Part model, mm, in its own coordinate system. Round coordinates to 2 decimals unless told otherwise and drop trailing zeros. Write each loop counter-clockwise with the first axis right and the second up, starting at its lowest first coordinate (ties: lowest second). Pieces come first, ordered by that corner, then holes. Notation, with made-up numbers: (78.25, 68) -> (121.25, 68) arc R26 cw to (121.25, 105) -> close; hole circle Ø6 at (63, 78.5). An arc over 180 degrees is marked (long way). Return JSON: item names as keys, results as strings. Group by question number.
(1) Saw through at B-B (x = 1.05). List the corners of the cut face in (y, z), plus the area to 3 significant figures.
(2) Drop flat-ended pins along their axis: pin 1 Ø1.7 at (x, y) = (-21, 1.5) entering from +Z; pin 2 Ø2.5 at (x, y) = (-16, 1) entering from -Z; pin 3 Ø5 at (y, z) = (5, 44) entering from -X. Give the stop position or say it passes through.
(3) Drill centre lines: L1, parallel to X at y = 1.25, z = 115.25; L2, parallel to X at y = 0.4, z = 115.25; L3, parallel to X at y = 7, z = 142.5. Where is each one in solid material? Low to high. Write a range as from..to.
(4) Saw through at A-A (y = 3.75). List the corners of the cut face in (x, z), plus the area to 3 significant figures.
(5) Saw through at C-C (z = 115.25). List the corners of the cut face in (x, y).
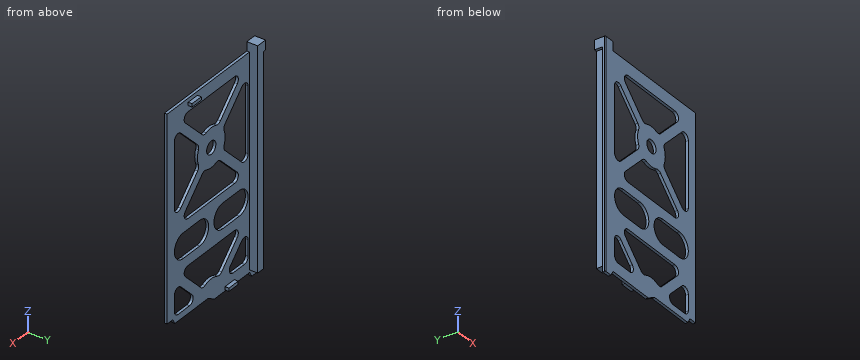
from build123d import *

# Parameters (mm, degrees)
SKETCH1_R           = 5
BOSS_EXTRUDE1_DEPTH = 2.1
SKETCH2_W           = 8.5
SKETCH2_H           = 170.25
BOSS_EXTRUDE2_DEPTH = 6.4
SKETCH3_W           = 162.8
SKETCH3_H           = 6.4
CUT_EXTRUDE1_DEPTH  = 2.1
SKETCH4_W           = 10
SKETCH4_H           = 2.5
BOSS_EXTRUDE3_DEPTH = 3
CHAMFER1_SIZE       = 0.5


with BuildPart() as part:
    # Sketch1 → Boss-Extrude1 (new body)
    with BuildSketch(Plane(origin=(0, 0, 0), x_dir=(1, 0, 0), z_dir=(0, 1, 0))):
        Polygon((-48.95, 0.55), (-48.95, -172.25), (-40.45, -172.25), (-40.45, -165.25), (48.95, -165.25), (48.95, -8), (42.85, -8), (40.540598923, -4), (4.514101615, -4), (-2.414101615, 0), (-40.640598923, 0), (-42.95, 4), (-48.95, 4), align=None)
        with BuildLine():
            Line((-13.76890063, -125.119153161), (-32.121572875, -143.471825407))
            ThreePointArc((-32.121572875, -143.471825407), (-36.480733729, -144.338916412), (-38.95, -140.643398282))
            Line((-38.95, -140.643398282), (-38.95, -89.856601718))
            ThreePointArc((-38.95, -89.856601718), (-36.480733729, -86.161083588), (-32.121572875, -87.028174593))
            Line((-32.121572875, -87.028174593), (-13.76890063, -105.380846839))
            ThreePointArc((-13.76890063, -105.380846839), (-12.679375, -107.403267629), (-12.882100859, -109.691532076))
            ThreePointArc((-12.882100859, -109.691532076), (-13.95, -115.25), (-12.882100859, -120.808467924))
            ThreePointArc((-12.882100859, -120.808467924), (-12.679375, -123.096732371), (-13.76890063, -125.119153161))
        make_face(mode=Mode.SUBTRACT)
        with BuildLine():
            ThreePointArc((-24.343398282, -155.25), (-28.038916412, -152.780733729), (-27.171825407, -148.421572875))
            Line((-27.171825407, -148.421572875), (-8.819153161, -130.06890063))
            ThreePointArc((-8.819153161, -130.06890063), (-6.796732371, -128.979375), (-4.508467924, -129.182100859))
            ThreePointArc((-4.508467924, -129.182100859), (1.05, -130.25), (6.608467924, -129.182100859))
            ThreePointArc((6.608467924, -129.182100859), (8.896732371, -128.979375), (10.919153161, -130.06890063))
            Line((10.919153161, -130.06890063), (29.271825407, -148.421572875))
            ThreePointArc((29.271825407, -148.421572875), (30.138916412, -152.780733729), (26.443398282, -155.25))
            Line((26.443398282, -155.25), (-24.343398282, -155.25))
        make_face(mode=Mode.SUBTRACT)
        with Locations((1.05, -115.25)):
            Circle(SKETCH1_R, mode=Mode.SUBTRACT)
        with BuildLine():
            Line((29.271825407, -82.078427125), (10.919153161, -100.43109937))
            ThreePointArc((10.919153161, -100.43109937), (8.896732371, -101.520625), (6.608467924, -101.317899141))
            ThreePointArc((6.608467924, -101.317899141), (1.05, -100.25), (-4.508467924, -101.317899141))
            ThreePointArc((-4.508467924, -101.317899141), (-6.796732371, -101.520625), (-8.819153161, -100.43109937))
            Line((-8.819153161, -100.43109937), (-27.171825407, -82.078427125))
            ThreePointArc((-27.171825407, -82.078427125), (-28.038916412, -77.719266271), (-24.343398282, -75.25))
            Line((-24.343398282, -75.25), (26.443398282, -75.25))
            ThreePointArc((26.443398282, -75.25), (30.138916412, -77.719266271), (29.271825407, -82.078427125))
        make_face(mode=Mode.SUBTRACT)
        with BuildLine():
            ThreePointArc((41.05, -140.643398282), (38.580733729, -144.338916412), (34.221572875, -143.471825407))
            Line((34.221572875, -143.471825407), (15.86890063, -125.119153161))
            ThreePointArc((15.86890063, -125.119153161), (14.779375, -123.096732371), (14.982100859, -120.808467924))
            ThreePointArc((14.982100859, -120.808467924), (16.05, -115.25), (14.982100859, -109.691532076))
            ThreePointArc((14.982100859, -109.691532076), (14.779375, -107.403267629), (15.86890063, -105.380846839))
            Line((15.86890063, -105.380846839), (34.221572875, -87.028174593))
            ThreePointArc((34.221572875, -87.028174593), (38.580733729, -86.161083588), (41.05, -89.856601718))
            Line((41.05, -89.856601718), (41.05, -140.643398282))
        make_face(mode=Mode.SUBTRACT)
        with BuildLine():
            ThreePointArc((-29.325, -67.25), (-38.95, -57.625), (-29.325, -48))
            Line((-29.325, -48), (-11.45, -48))
            ThreePointArc((-11.45, -48), (-1.825, -57.625), (-11.45, -67.25))
            Line((-11.45, -67.25), (-29.325, -67.25))
        make_face(mode=Mode.SUBTRACT)
        with BuildLine():
            ThreePointArc((-38.95, -13), (-37.778427125, -10.171572875), (-34.95, -9))
            Line((-34.95, -9), (-22.556601718, -9))
            ThreePointArc((-22.556601718, -9), (-18.861083588, -11.469266271), (-19.728174593, -15.828427125))
            Line((-19.728174593, -15.828427125), (-32.121572875, -28.221825407))
            ThreePointArc((-32.121572875, -28.221825407), (-36.480733729, -29.088916412), (-38.95, -25.393398282))
            Line((-38.95, -25.393398282), (-38.95, -13))
        make_face(mode=Mode.SUBTRACT)
        with BuildLine():
            ThreePointArc((13.55, -67.25), (3.925, -57.625), (13.55, -48))
            Line((13.55, -48), (31.425, -48))
            ThreePointArc((31.425, -48), (41.05, -57.625), (31.425, -67.25))
            Line((31.425, -67.25), (13.55, -67.25))
        make_face(mode=Mode.SUBTRACT)
        with BuildLine():
            ThreePointArc((-24.343398282, -40), (-28.038916412, -37.530733729), (-27.171825407, -33.171572875))
            Line((-27.171825407, -33.171572875), (-10.202325554, -16.202073022))
            ThreePointArc((-10.202325554, -16.202073022), (-8.02311566, -15.083537139), (-5.600446128, -15.445131695))
            ThreePointArc((-5.600446128, -15.445131695), (1.05, -17), (7.700446128, -15.445131695))
            ThreePointArc((7.700446128, -15.445131695), (10.12311566, -15.083537139), (12.302325554, -16.202073022))
            Line((12.302325554, -16.202073022), (29.271825407, -33.171572875))
            ThreePointArc((29.271825407, -33.171572875), (30.138916412, -37.530733729), (26.443398282, -40))
            Line((26.443398282, -40), (-24.343398282, -40))
        make_face(mode=Mode.SUBTRACT)
        with BuildLine():
            ThreePointArc((37.05, -9), (39.878427125, -10.171572875), (41.05, -13))
            Line((41.05, -13), (41.05, -25.393398282))
            ThreePointArc((41.05, -25.393398282), (38.580733729, -29.088916412), (34.221572875, -28.221825407))
            Line((34.221572875, -28.221825407), (21.828174593, -15.828427125))
            ThreePointArc((21.828174593, -15.828427125), (20.961083588, -11.469266271), (24.656601718, -9))
            Line((24.656601718, -9), (37.05, -9))
        make_face(mode=Mode.SUBTRACT)
    extrude(amount=BOSS_EXTRUDE1_DEPTH)

    # Sketch2 → Boss-Extrude2 (add)
    with BuildSketch(Plane(origin=(0, 2.1, 0), x_dir=(1, 0, 0), z_dir=(0, 1, 0))):
        with Locations((-44.7, -87.125)):
            Rectangle(SKETCH2_W, SKETCH2_H)
    extrude(amount=BOSS_EXTRUDE2_DEPTH)

    # Sketch3 → Cut-Extrude1 (cut)
    with BuildSketch(Plane.ZY.offset(48.95)):
        with Locations((83.4, 5.3)):
            Rectangle(SKETCH3_W, SKETCH3_H)
    extrude(amount=-CUT_EXTRUDE1_DEPTH, mode=Mode.SUBTRACT)

    # Sketch4 → Boss-Extrude3 (add)
    with BuildSketch(Plane(origin=(0, 2.1, 0), x_dir=(1, 0, 0), z_dir=(0, 1, 0))):
        with Locations((-18.95, -2)):
            Rectangle(SKETCH4_W, SKETCH4_H)
        with Locations((21.05, -161)):
            Rectangle(SKETCH4_W, SKETCH4_H)
    extrude(amount=BOSS_EXTRUDE3_DEPTH)

    # Chamfer1
    chamfer1_edges = [part.edges().sort_by_distance(p)[0] for p in [
        (-48.95, 0, 84.125),
    ]]
    chamfer(chamfer1_edges, length=CHAMFER1_SIZE)


solid = part.part
Computed values:
{
 "1": {"outline": "(0, 2) -> (2.1, 2) -> (2.1, 17) -> (0, 17) -> close; (0, 40) -> (2.1, 40) -> (2.1, 75.25) -> (0, 75.25) -> close; (0, 100.25) -> (2.1, 100.25) -> (2.1, 110.25) -> (0, 110.25) -> close; (0, 120.25) -> (2.1, 120.25) -> (2.1, 130.25) -> (0, 130.25) -> close; (0, 155.25) -> (2.1, 155.25) -> (2.1, 165.25) -> (0, 165.25) -> close", "area": "169 mm2"},
 "2": {"pin 1": "z = 165.25", "pin 2": "z = 0", "pin 3": "x = -46.85"},
 "3": {"L1": "-48.95..-38.95, -13.95..-3.95, 6.05..16.05, 41.05..48.95", "L2": "-48.85..-38.95, -13.95..-3.95, 6.05..16.05, 41.05..48.95", "L3": "-46.85..-40.45"},
 "4": {"outline": "(-48.95, 164.8) -> (-46.85, 164.8) -> (-46.85, 2) -> (-40.45, 2) -> (-40.45, 172.25) -> (-48.95, 172.25) -> close; (-23.95, 0.75) -> (-13.95, 0.75) -> (-13.95, 3.25) -> (-23.95, 3.25) -> close; (16.05, 159.75) -> (26.05, 159.75) -> (26.05, 162.25) -> (16.05, 162.25) -> close", "area": "1,160 mm2"},
 "5": {"outline": "(-48.95, 0.5) -> (-48.45, 0) -> (-38.95, 0) -> (-38.95, 2.1) -> (-40.45, 2.1) -> (-40.45, 8.5) -> (-46.85, 8.5) -> (-46.85, 2.1) -> (-48.95, 2.1) -> close; (-13.95, 0) -> (-3.95, 0) -> (-3.95, 2.1) -> (-13.95, 2.1) -> close; (6.05, 0) -> (16.05, 0) -> (16.05, 2.1) -> (6.05, 2.1) -> close; (41.05, 0) -> (48.95, 0) -> (48.95, 2.1) -> (41.05, 2.1) -> close"}
}
